Geometry: final body of the model. Coordinates: model frame, mm. A direction names the side the tool comes from. Give positions to 0.01 mm unless a question says otherwise; leave off trailing zeros. Loops run counter-clockwise (first coordinate to the right, second up) from the corner with the lowest first, then second, coordinate; pieces in that order, holes last. Notation, with made-up numbers: M 87.25,56 L 118.25,56 A19 ccw 118.25,73 Z; hole C 43.5,25.25 d2. An arc over 180 degrees is marked long. Put each result on its own line as item: value.
Autodesk Inventor part; units mm, degrees
ref_plane "YZ Plane" through (0, 0, 0) normal (1, 0, 0) x (0, 1, 0)
ref_plane "XZ Plane" through (0, 0, 0) normal (0, 1, 0) x (-1, 0, 0)
ref_plane "XY Plane" through (0, 0, 0) normal (0, 0, 1) x (1, 0, 0)
sketch "Sketch1" plane through (0, 0, 0) normal (0, 1, 0) x (-1, 0, 0)
  line L0 (0.1637, 10.9307) -> (0.1637, -2.5693)
  line L1 (0.1637, -59.5693) -> (0.1637, -73.0693)
  line L2 (0.1637, -2.5693) -> (15.1637, -2.5693)
  line L3 (0.1637, -59.5693) -> (15.1637, -59.5693)
  line L4 (15.1637, -2.5693) -> (23.6637, -11.0693)
  line L5 (15.1637, -59.5693) -> (23.6637, -51.0693)
  line L6 (23.6637, -11.0693) -> (23.6637, -51.0693)
  line L7 (4.1637, -73.0693) -> (4.1637, -63.5693)
  line L8 (4.1637, -63.5693) -> (16.8205, -63.5693)
  line L9 (16.8205, -63.5693) -> (27.6637, -52.7262)
  line L10 (27.6637, -52.7262) -> (27.6637, -9.4125)
  line L11 (27.6637, -9.4125) -> (16.8205, 1.4307)
  line L12 (16.8205, 1.4307) -> (4.1637, 1.4307)
  line L13 (4.1637, 1.4307) -> (4.1637, 10.9307)
  line L14 (4.1637, 10.9307) -> (0.1637, 10.9307)
  line L15 (4.1637, -73.0693) -> (0.1637, -73.0693)
  point P0 (0, 0)
  point P1 (0.1637, 4.1807)
  dimension "d5" = 13.5
  dimension "d6" = 13.5
  dimension "d98" = 0
  dimension "d100" = 15
  dimension "d101" = 15
  dimension "d103" = 135
  dimension "d104" = 135
  dimension "d106" = 23.5
  dimension "d107" = 4
  dimension "d111" = 84
extrude "Extrusion1" add sketch "Sketch1" along normal blind 26
sketch "Sketch2" plane through (-0.1637, 0, 10.9307) normal (1, 0, 0) x (0, 0, -1)
  circle A0 centre (6.5, 13) radius 2.25
  line L0 (0, 0) -> (0, 26)
  line L1 (0, 0) -> (13.5, 0)
  circle A1 centre (77.5, 13) radius 2.25
  point P0 (10.9307, 0)
  dimension "d23" = 4.5
  dimension "d29" = 6.5
  dimension "d30" = 13
  dimension "d93" = 71
extrude "Extrusion2" cut sketch "Sketch2" against normal blind 10
sketch "Sketch7" plane through (-27.6637, 0, -52.7262) normal (-1, 0, 0) x (0, 0, 1)
  circle A0 centre (21.6569, 13) radius 6
  line L0 (63.6569, 0) -> (63.6569, 26)
  line L1 (0, 0) -> (43.3137, 0)
  point P0 (52.7262, 0)
  point P1 (21.6569, 0)
  dimension "d108" = 12
  dimension "d109" = 42
  dimension "d110" = 13
extrude "Extrusion7" cut sketch "Sketch7" against normal blind 10
sketch "Sketch8" plane through (-27.6637, 0, -52.7262) normal (-1, 0, 0) x (0, 0, 1)
  circle A0 centre (21.6569, 13) radius 6
  circle A1 centre (21.6569, 13) radius 18.35
  circle A2 centre (38.4042, 5.5) radius 2.5
  line L0 (0, 0) -> (43.3137, 0)
  circle A3 centre (4.9095, 20.5) radius 2.5
  point P0 (52.7262, 0)
  dimension "d114" = 36.7
  dimension "d115" = 5
  dimension "d116" = 5.5
  dimension "d119" = 360
extrude "Extrusion8" cut sketch "Sketch8" against normal blind 10 contours A3 A1 | A1 A3 | A2 A1 | A1 A2
sketch "Sketch9" plane through (-4.1637, 0, 1.4307) normal (-1, 0, 0) x (0, 0, 1)
  circle A0 centre (3, 13.0738) radius 4
  circle A1 centre (-68, 13.0738) radius 4
  point P0 (-1.4307, 0)
  dimension "d123" = 8
  dimension "d124" = 8
extrude "Extrusion9" cut sketch "Sketch9" along normal blind 4
equation "\"d5\" = d6"
equation "\"d29\" = -0.5 * d33 + 0.5 * d17"
equation "\"d30\" = 0.5 * d20"
properties part number "Pulley Bearing Support.-3"
Item 1: Section D-D on y = 20.5. Output: boundary loops of the cut face in (x, z), then the cut area to 3 significant figures.
Output values:
outline: M -27.66,-52.73 L -16.82,-63.57 L -4.16,-63.57 L -4.16,-73.07 L -0.16,-73.07 L -0.16,-59.57 L -15.16,-59.57 L -23.66,-51.07 L -23.66,-50.32 L -27.66,-50.32 Z; M -27.66,-45.32 L -23.66,-45.32 L -23.66,-11.07 L -15.16,-2.57 L -0.16,-2.57 L -0.16,10.93 L -4.16,10.93 L -4.16,1.43 L -16.82,1.43 L -27.66,-9.41 Z
area: 459 mm²
Item 2: Pin query (flat end, axial travel): pin 1 Ø8.5 at (y, z) = (17, -65.5) entering from -X; pin 2 Ø11.5 at (y, z) = (19, 5.5) entering from -X; pin 3 Ø8 at (y, z) = (14.5, -46.5) entering from +X. Return the tip coordinate at first contact, or that it passes through.
Output values:
pin 1: x = -19.14
pin 2: x = -18.5
pin 3: x = -23.66
Item 3: Mould query, pull axis X, two halves, no side actions, for faces 6 (the flat face through (-22.32, 12.82, -4.07)), 7 (the cylindrical face through (-6.14, 13.03, 0.43)), 8 (the flat face through (-24, 26, -31)), 9 (the flat face through (-19.354, 12.818, -55.379)). Classes: pulls with the +X half, pulls with the -X half, needs draft (parallel to the pull), parting line crosses it, or undercut.
Output values:
face 6: pulls with the -X half
face 7: undercut
face 8: needs draft
face 9: pulls with the +X half
Item 4: Section C-C on z = -26.5. Output: boundary loops of the cut face in (x, y).
Output values:
outline: M -27.66,0 L -23.66,0 L -23.66,9.11 L -27.66,9.11 Z; M -27.66,16.89 L -23.66,16.89 L -23.66,26 L -27.66,26 Z
Item 5: Set-up query: faces 1 (the flat face through (-8, 13, -59.569)), 2 (the flat face through (-22.17, 12.82, -58.22)), 3 (the cylindrical face through (-6.14, 13.11, -62.57)), 4 (the flat face through (-11, 13, 1.431)), 5 (the flat face through (-2, 13, 10.931)). Return all of +Z, -Z, +X, -X, +Y, -Y with unobstructed straight access to the full face (end or side cutting, diameter ignored); none if empty.
Output values:
face 1: +X, +Y, -Y
face 2: -Z, -X, +Y, -Y
face 3: -Z
face 4: +Z, -X, +Y, -Y
face 5: +Z, +X, -X, +Y, -Y
Item 6: Section A-A on x = -3.25. Output: boundary loops of the cut face in (y, z), then the cut area to 3 significant figures.
Output values:
outline: M 0,-73.07 L 26,-73.07 L 26,-59.57 L 0,-59.57 Z; M 0,-2.57 L 26,-2.57 L 26,10.93 L 0,10.93 Z; hole C 13,-66.57 d4.5; hole C 13,4.43 d4.5
area: 670 mm²
Item 7: Section B-B on x = -13.5. Output: boundary loops of the cut face in (y, z).
Output values:
outline: M 0,-63.57 L 26,-63.57 L 26,-59.57 L 0,-59.57 Z; M 0,-2.57 L 26,-2.57 L 26,1.43 L 0,1.43 Z
Item 8: Line query: probe 1 along Z at (x, y) = (-11, 23.25); probe 2 along Z at (x, y) = (-1.5, 21); probe 3 along X at (y, z) = (2.25, -15.5). Output: solid intervals per line, ascending. Write a range as [from, to].
Output values:
probe 1: [-63.57, -59.57], [-2.57, 1.43]
probe 2: [-73.07, -59.57], [-2.57, 10.93]
probe 3: [-27.66, -23.66]
